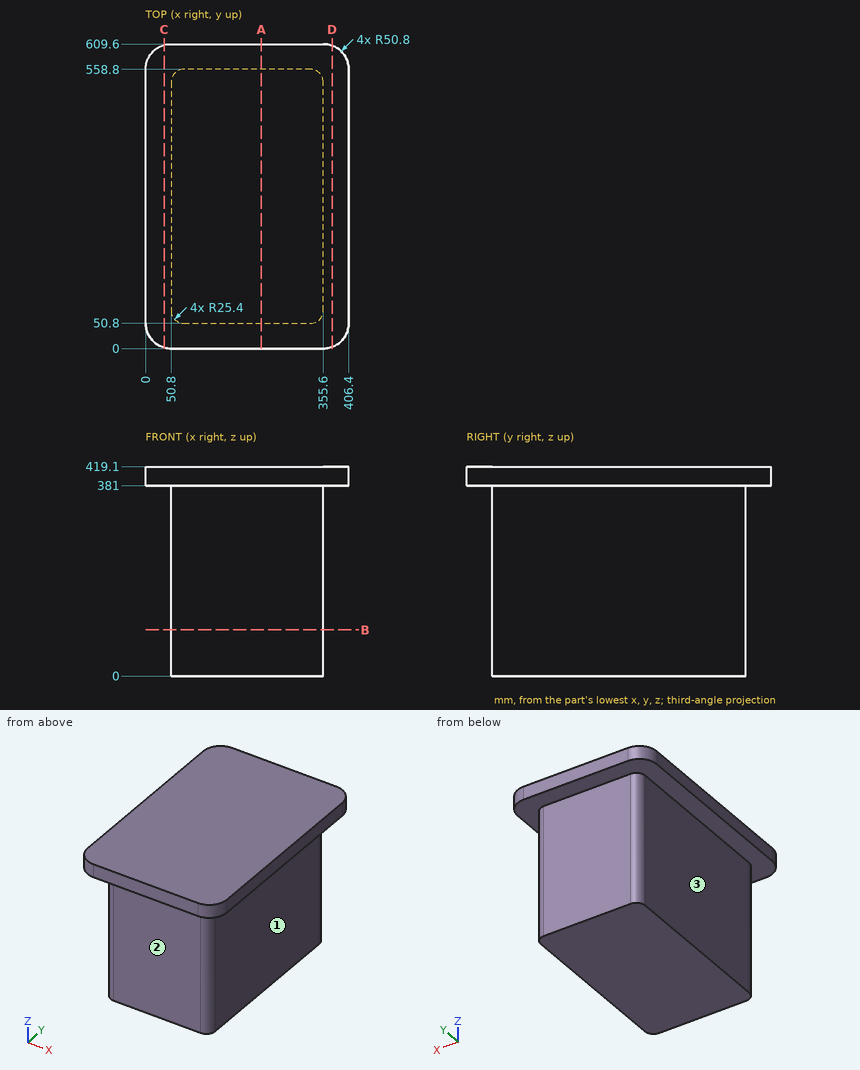
Print and shaded views of the part. All mm, measured from the part's lowest x, y and z. A direction names the side the tool comes from. Coordinates: 2 decimals unless noted, no trailing zeros. Order: outer loops, then holes, each group sorted by start corner. A loop starts at its lowest first (then second) coordinate and runs counter-clockwise, first axis right, second up. Notation, with made-up numbers: (81, 65.25) -> (118, 65.25) arc R11 cw to (118, 86.25) -> close; hole circle Ø3 at (24.25, 46.5). An arc over 180 degrees is marked (long way). Answer as a JSON object with one key per item and string values. Group by question number.
1) Cut at C-C, the plane x = 37. Write the cut outline in (y, z).
2) Cut at D-D, the plane x = 373. Write the cut outline in (y, z), then the cut area to 3 significant figures.
3) Drill centre lines: L1, parallel to X at y = 224.5, z = 300; L2, parallel to Z at x = 369.5, y = 474; L3, parallel to Y at x = 254.5, z = 29.5. Where is each one in solid material? Low to high.
4) Cut at A-A, the plane x = 231.5. Write the cut outline in (y, z), then the cut area to 3 significant figures.
5) Which spindle directions (+Z, -Z, +X, -X, +Y, -Y) get a long thin tool onto all of the face, cutting with end or side? Do the marked faces 1, 2 and 3. Say none if no direction does.
6) Cut at B-B, the plane z = 92.5. Write the cut outline in (x, y).
7) Flat gauge pins, fed straight in: pin 1 (8 mm diameter, centred on x = 263.5, y = 480, fed in from -Z); pin 2 (2 mm diameter, centred on x = 171, z = 373.5, fed in from +Y); pin 3 (2 mm diameter, centred on y = 240.5, z = 48, fed in from -X); pin 4 (8 mm diameter, centred on y = 428.5, z = 277.5, fed in from +X). Where does each tip first touch, or does it go through?
Check values:
{
 "1": {"outline": "(1.91, 381) -> (607.69, 381) -> (607.69, 419.1) -> (1.91, 419.1) -> close"},
 "2": {"outline": "(3.07, 381) -> (606.53, 381) -> (606.53, 419.1) -> (3.07, 419.1) -> close", "area": "23,000 mm²"},
 "3": {"L1": "x = 50.8 to 355.6", "L2": "z = 381 to 419.1", "L3": "y = 50.8 to 558.8"},
 "4": {"outline": "(0, 381) -> (50.8, 381) -> (50.8, 0) -> (558.8, 0) -> (558.8, 381) -> (609.6, 381) -> (609.6, 419.1) -> (0, 419.1) -> close", "area": "217,000 mm²"},
 "5": {"face 1": "-Z, +X, +Y, -Y", "face 2": "-Z, +X, -X, -Y", "face 3": "-Z, -X, +Y, -Y"},
 "6": {"outline": "(50.8, 76.2) arc R25.4 ccw to (76.2, 50.8) -> (330.2, 50.8) arc R25.4 ccw to (355.6, 76.2) -> (355.6, 533.4) arc R25.4 ccw to (330.2, 558.8) -> (76.2, 558.8) arc R25.4 ccw to (50.8, 533.4) -> close"},
 "7": {"pin 1": "stops at z = 0", "pin 2": "stops at y = 558.8", "pin 3": "stops at x = 50.8", "pin 4": "stops at x = 355.6"}
}
